For this review, take the finished solid that the model builds, in its own axes (mm). A direction names the side the tool comes from. Give positions to 0.01 mm unless a question says otherwise; leave off trailing zeros. Loops run counter-clockwise (first coordinate to the right, second up) from the corner with the lowest first, then second, coordinate; pieces in that order, holes last.
```python
from build123d import *

# Parameters (mm, degrees)
SKETCH_1_R               = 11.5
EXTRUDE_1_DEPTH          = 0.5
SKETCH_2_R               = 9.295
EXTRUDE_2_DEPTH          = 11
CUT_EXTRUDE_3_DEPTH      = 11
SKETCH_3_R               = 11.5
EXTRUDE_3_DEPTH          = 1
SKETCH_6_R               = 4
CUT_EXTRUDE_2_DEPTH      = 1
CUT_EXTRUDE_2_DEPTH_BACK = 14
PATTERN_CIRCULAR_2_COUNT = 30


with BuildPart() as part:
    # 草圖1 → 填料-伸長1 (new body, symmetric)
    with BuildSketch(Plane.XY):
        Circle(SKETCH_1_R)
    extrude(amount=EXTRUDE_1_DEPTH, both=True)

    # 草圖2 → 填料-伸長2 (add)
    with BuildSketch(Plane.XY.offset(0.5)):
        Circle(SKETCH_2_R)
    extrude(amount=EXTRUDE_2_DEPTH)

    # 草圖7 → 除料-伸長3 (cut)
    with BuildSketch(Plane.XY.offset(11.5)):
        with BuildLine():
            ThreePointArc((-0.599687408, 9.27563475), (0, 8.695), (0.599687408, 9.27563475))
            ThreePointArc((0.599687408, 9.27563475), (0, 9.295), (-0.599687408, 9.27563475))
        make_face()
    cut_extrude_3 = extrude(amount=-CUT_EXTRUDE_3_DEPTH, mode=Mode.SUBTRACT)

    # 草圖3 → 填料-伸長3 (add)
    with BuildSketch(Plane.XY.offset(11.5)):
        Circle(SKETCH_3_R)
    extrude(amount=EXTRUDE_3_DEPTH)

    # 草圖6 → 除料-伸長2 (cut, two sides)
    with BuildSketch(Plane(origin=(0, 0, -0.5), x_dir=(-1, 0, 0), z_dir=(0, 0, -1))) as cut_extrude_2_sk:
        Circle(SKETCH_6_R)
    extrude(amount=CUT_EXTRUDE_2_DEPTH, mode=Mode.SUBTRACT)
    extrude(cut_extrude_2_sk.sketch, amount=-CUT_EXTRUDE_2_DEPTH_BACK, mode=Mode.SUBTRACT)

    # 環狀複製排列2: 除料-伸長3 ×30 about axis
    pattern_circular_2_axis = Axis((0, 0, 0), (0, 0, 1))
    for i in range(1, PATTERN_CIRCULAR_2_COUNT):
        add(cut_extrude_3.rotate(pattern_circular_2_axis, i * 360 / PATTERN_CIRCULAR_2_COUNT), mode=Mode.SUBTRACT)


solid = part.part
```
Q1. Machinability: for faces 1 (the cylindrical face through (0.867, -3.905, 5.909)), 2 (the cylindrical face through (-3.52, -7.95, 6.08)), 3 (the cylindrical face through (0.013, -8.695, 6.077)), which of the approach directions +Z, -Z, +X, -X, +Y, -Y give a long, thin tool a straight path to every point of the face, cutting with its end or side? Answer none if there is none.
Answers:
face 1: +Z, -Z
face 2: none
face 3: -Y
Q2. Mouldability with a two-part tool opening along Y and no side actions: class faces 4 (the cylindrical face through (-1.5, 11.4, 12)), 5 (the cylindrical face through (-0.013, 8.695, 6.077)), 6 (the cylindrical face through (8.266, 2.699, 6.077)) as +Y half, -Y half, draft (parallel to the pull), parting line (faces both ways), or undercut.
Answers:
face 4: parting line
face 5: +Y half
face 6: undercut
Q3. For pin 1 Ø5 at (x, y) = (0, 0) entering from -Z; pin 2 Ø3 at (y, z) = (8, 4.5) entering from -X; pin 3 Ø1.5 at (x, z) = (-2.5, 6) entering from +Y; pin 4 Ø6 at (y, z) = (0, 8) entering from +X (3 decimals), all flat-tipped, find the tip position at first contact; note any pin that passes through.
Answers:
pin 1: passes through
pin 2: stops at x = -6.49
pin 3: stops at y = 8.95
pin 4: stops at x = 9.295
Q4. For probe 1 along Y at (x, z) = (0, 2.5) (3 decimals); probe 2 along Z at (x, y) = (-9, -5.5); probe 3 along Y at (x, z) = (5.5, 5), list the stretches that pass through material, from the lowest coordinate up.
Answers:
probe 1: y = -8.695 to -4, 4 to 8.695
probe 2: z = -0.5 to 0.5, 11.5 to 12.5
probe 3: y = -6.92 to 6.92
Q5. Consider section A-A on x = 0. Give the boundary of the cut face in (y, z) (3 decimals).
Answers:
outline: (-11.5, -0.5) - (-4, -0.5) - (-4, 12.5) - (-11.5, 12.5) - (-11.5, 11.5) - (-8.695, 11.5) - (-8.695, 0.5) - (-11.5, 0.5) - close; (4, -0.5) - (11.5, -0.5) - (11.5, 0.5) - (8.695, 0.5) - (8.695, 11.5) - (11.5, 11.5) - (11.5, 12.5) - (4, 12.5) - close
Q6. Consider section B-B on y = 0. Give the boundary of the cut face in (x, z) (3 decimals), plus the area to 3 significant figures.
Answers:
outline: (-11.5, -0.5) - (-4, -0.5) - (-4, 12.5) - (-11.5, 12.5) - (-11.5, 11.5) - (-9.295, 11.5) - (-9.295, 0.5) - (-11.5, 0.5) - close; (4, -0.5) - (11.5, -0.5) - (11.5, 0.5) - (9.295, 0.5) - (9.295, 11.5) - (11.5, 11.5) - (11.5, 12.5) - (4, 12.5) - close
area: 146 mm2
